Source: CAD feature listing. Evaluate the final solid. Frame: model axes, mm. Give positions to 0.01 mm unless a question says otherwise; leave off trailing zeros. Order: outer loops, then holes, each group sorted by start corner. A loop starts at its lowest first (then second) coordinate and runs counter-clockwise, first axis right, second up.
1) Material intervals for line 1 (Y direction, x = 9.75, z = 160); line 2 (Y direction, x = 11.5, z = 147); line 3 (Y direction, x = 11.75, z = 247), sorted ascending.
2) Section A-A, the plane x = 10. Give the number of separate pieces and of enclosed holes in the cut face, plus the area to 3 significant figures.
3) First-contact query: P1, Ø1.5, axis at x = 5.5, y = 84, coming from the +Z side; P2, Ø6, axis at x = 3, z = 185, coming from the +Y side; P3, Ø5, axis at x = 8.5, z = 216.5, coming from the +Y side. Flat tips, straight axial feed; report the tip coordinate or a pass-through.
4) Section C-C, the plane y = 89. Return loops of the section in (x, z).
5) Draft query along Y for faces 1 (the face through (6.26, 58.27, 205.66)), 2 (the face through (6.261, -17.222, 284.265)), 3 (the face through (6.261, -10.796, 282.577)). Return one class per face: released by +Y, released by -Y, zero draft, split by the parting line, or undercut.
6) Section B-B, the plane z = 225. Return loops of the section in (x, y).
```python
from build123d import *

# Parameters (mm, degrees)
F0_R     = 4.7625
F1_DEPTH = 12.7


# Not quite as in the source:
# - a feature names something its author has since deleted; it is built from what else it names


with BuildPart() as f1:
    # F0 (on Right) → F1 (new body)
    with BuildSketch(Plane.YZ):
        with BuildLine():
            ThreePointArc((135.0932664818, 138.7993858615), (134.1614165409, 152.23749978), (147.5995304594, 153.1693497209))
            Line((147.5995304594, 153.1693497209), (-3.9226998699, 285.0400370456))
            ThreePointArc((-3.9226998699, 285.0400370456), (-1.5073052482, 281.8024937035), (-0.6508318587, 277.8550551158))
            ThreePointArc((-0.6508318587, 277.8550551158), (-6.2283932711, 269.1865285054), (-16.4289638475, 270.6700731861))
            Line((-16.4289638475, 270.6700731861), (135.0932664818, 138.7993858615))
        make_face()
        with BuildLine():
            ThreePointArc((-0.6508318587, 277.8550551158), (-1.5073052482, 281.8024937035), (-3.9226998699, 285.0400370456))
            ThreePointArc((-3.9226998699, 285.0400370456), (-17.3608137885, 284.1081871047), (-16.4289638475, 270.6700731861))
            ThreePointArc((-16.4289638475, 270.6700731861), (-6.2283932711, 269.1865285054), (-0.6508318587, 277.8550551158))
        make_face()
        with Locations((-10.1758318587, 277.8550551158)):
            Circle(F0_R, mode=Mode.SUBTRACT)
        with BuildLine():
            ThreePointArc((135.0932664818, 138.7993858615), (145.2938370582, 137.3158411807), (150.8713984706, 145.9843677912))
            ThreePointArc((150.8713984706, 145.9843677912), (150.0149250811, 149.9318063789), (147.5995304594, 153.1693497209))
            ThreePointArc((147.5995304594, 153.1693497209), (134.1614165409, 152.23749978), (135.0932664818, 138.7993858615))
        make_face()
        with Locations((141.3463984706, 145.9843677912)):
            Circle(F0_R, mode=Mode.SUBTRACT)
    extrude(amount=F1_DEPTH)


solid = f1.part
```
From the geometry:
1. line 1: y = 110.73 to 139.75
1. line 2: y = 125.67 to 136.69, 146 to 150.82
1. line 3: y = 10.77 to 39.79
2. separate pieces: 1
2. enclosed holes: 2
2. area: 3,970 mm2
3. P1: stops at z = 209.17
3. P2: stops at y = 114.47
3. P3: stops at y = 77.7
4. outline: (0, 178.91) - (12.7, 178.91) - (12.7, 204.17) - (0, 204.17) - close
5. face 1: released by -Y
5. face 2: split by the parting line
5. face 3: undercut
6. outline: (0, 36.05) - (12.7, 36.05) - (12.7, 65.06) - (0, 65.06) - close
